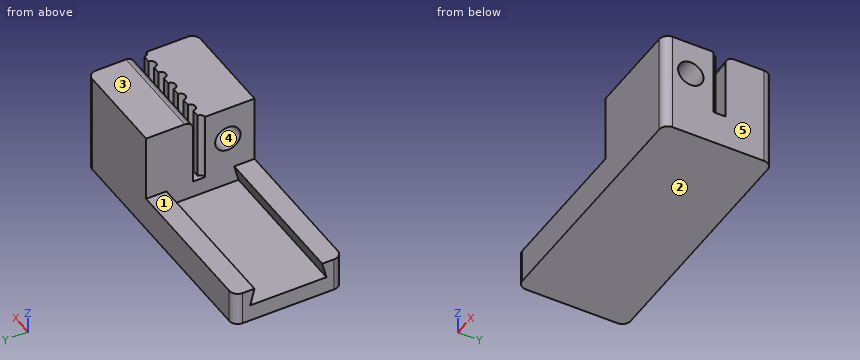
```python
from build123d import *

# Parameters (mm, degrees)
BOSS_EXTRUDE1_DEPTH = 12
CUT_EXTRUDE1_DEPTH  = 8
FILLET1_R           = 1
CUT_EXTRUDE3_DEPTH  = 18
SKETCH6_R           = 1.5
CUT_EXTRUDE2_DEPTH  = 12


with BuildPart() as part:
    # Sketch4 → Boss-Extrude1 (new body)
    with BuildSketch(Plane.XY):
        with BuildLine():
            Line((12, 1.1), (12, 11.9))
            ThreePointArc((12, 11.9), (11.707106781, 12.607106781), (11, 12.9))
            Line((11, 12.9), (-17, 12.9))
            ThreePointArc((-17, 12.9), (-17.707106781, 12.607106781), (-18, 11.9))
            Line((-18, 11.9), (-18, 1.1))
            ThreePointArc((-18, 1.1), (-17.707106781, 0.392893219), (-17, 0.1))
            Line((-17, 0.1), (11, 0.1))
            ThreePointArc((11, 0.1), (11.707106781, 0.392893219), (12, 1.1))
        make_face()
    extrude(amount=BOSS_EXTRUDE1_DEPTH)

    # Sketch5 → Cut-Extrude1 (cut)
    with BuildSketch(Plane.XY.offset(12)):
        with BuildLine():
            Line((11.445, 6.5), (10.555, 6.5))
            ThreePointArc((10.555, 6.5), (10, 5.945), (9.445, 6.5))
            Line((9.445, 6.5), (8.555, 6.5))
            ThreePointArc((8.555, 6.5), (8, 5.945), (7.445, 6.5))
            Line((7.445, 6.5), (6.555, 6.5))
            ThreePointArc((6.555, 6.5), (6, 5.945), (5.445, 6.5))
            Line((5.445, 6.5), (4.555, 6.5))
            ThreePointArc((4.555, 6.5), (4, 5.945), (3.445, 6.5))
            Line((3.445, 6.5), (2.555, 6.5))
            ThreePointArc((2.555, 6.5), (2, 5.945), (1.445, 6.5))
            Line((1.445, 6.5), (0.555, 6.5))
            ThreePointArc((0.555, 6.5), (0.392444264, 6.107555736), (0, 5.945))
            Line((0, 5.945), (0, 7.345))
            Line((0, 7.345), (12, 7.345))
            Line((12, 7.345), (12, 5.945))
            ThreePointArc((12, 5.945), (11.607555736, 6.107555736), (11.445, 6.5))
        make_face()
    extrude(amount=-CUT_EXTRUDE1_DEPTH, mode=Mode.SUBTRACT)

    # Fillet1
    fillet1_edges = [part.edges().sort_by_distance(p)[0] for p in [
        (6, 7.345, 12),
    ]]
    fillet(fillet1_edges, radius=FILLET1_R)

    # Sketch7 → Cut-Extrude3 (cut)
    with BuildSketch(Plane.ZY.offset(18)):
        Polygon((4, 10.5), (4, 12.9), (12, 12.9), (12, 0.1), (4, 0.1), (4, 2.5), (2, 2), (2, 11), align=None)
    extrude(amount=-CUT_EXTRUDE3_DEPTH, mode=Mode.SUBTRACT)

    # Sketch6 → Cut-Extrude2 (cut)
    with BuildSketch(Plane.ZY.offset(-12)):
        with Locations((8, 3.25)):
            Circle(SKETCH6_R)
    extrude(amount=CUT_EXTRUDE2_DEPTH, mode=Mode.SUBTRACT)


solid = part.part
```
Model file for the job. Use its own axes, mm. Face numbers are marked on the shaded views. A direction names the side the tool comes from. Give positions to 0.01 mm unless a question says otherwise; leave off trailing zeros. Order: outer loops, then holes, each group sorted by start corner. A loop starts at its lowest first (then second) coordinate and runs counter-clockwise, first axis right, second up.
1) Mould opens along Z. For the marked faces 3, 4 and 5 say: +Z half, -Z half, draft (parallel to the pull), parting line (faces both ways), or undercut.
2) Saw through at D-D, the plane x = 4. Write the cut outline in (y, z) (3 decimals).
3) Saw through at A-A, the plane y = 3.25. Write the cut outline in (x, z), then the cut area to 3 significant figures.
4) Saw through at C-C, the plane z = 10.5. Write the cut outline in (x, y) (3 decimals).
5) Pin check, flat tips, straight feed: pin 1 (3.5 mm diameter, centred on y = 3.25, z = 8, fed in from -X); pin 2 (2.5 mm diameter, centred on x = -9, y = 1.5, fed in from +Z); pin 3 (3 mm diameter, centred on x = -1.5, y = 8, fed in from -Z). Stop position of each tip, or through.
6) Wall check: probe 1 along Y at (x, z) = (6, 8) (3 decimals); probe 2 along Z at (x, y) = (9.5, 8.25). Give the ranges that are in metal, low to high.
7) Saw through at B-B, the plane z = 8. Write the cut outline in (x, y) (3 decimals), then the cut area to 3 significant figures.
8) 3-axis set-ups, long thin cutter, end or side, ignore diameter. For the marked faces 1 and 2: which of +Z, -Z, +X, -X, +Y, -Y reach the whole face in a straight line?
Computed:
1. face 3: +Z half
1. face 4: undercut
1. face 5: draft
2. outline: (0.1, 0) - (12.9, 0) - (12.9, 12) - (8.345, 12) arc R1 ccw to (7.345, 11) - (7.345, 4) - (5.945, 4) - (5.945, 12) - (0.1, 12) - close; hole circle Ø3 at (3.25, 8)
3. outline: (-18, 0) - (12, 0) - (12, 6.5) - (0, 6.5) - (0, 2) - (-18, 2) - close; (0, 9.5) - (12, 9.5) - (12, 12) - (0, 12) - close
3. area: 144 mm2
4. outline: (0, 0.1) - (11, 0.1) arc R1 ccw to (12, 1.1) - (12, 5.945) arc R0.555 cw to (11.445, 6.5) - (10.555, 6.5) arc R0.555 cw to (9.445, 6.5) - (8.555, 6.5) arc R0.555 cw to (7.445, 6.5) - (6.555, 6.5) arc R0.555 cw to (5.445, 6.5) - (4.555, 6.5) arc R0.555 cw to (3.445, 6.5) - (2.555, 6.5) arc R0.555 cw to (1.445, 6.5) - (0.555, 6.5) arc R0.555 cw to (0, 5.945) - close; (0, 7.345) - (12, 7.345) - (12, 11.9) arc R1 ccw to (11, 12.9) - (0, 12.9) - close
5. pin 1: stops at x = 0
5. pin 2: stops at z = 4
5. pin 3: stops at z = 0
6. probe 1: y = 0.1 to 1.75, 4.75 to 5.945, 7.345 to 12.9
6. probe 2: z = 0 to 12
7. outline: (0, 0.1) - (11, 0.1) arc R1 ccw to (12, 1.1) - (12, 1.75) - (0, 1.75) - close; (0, 4.75) - (12, 4.75) - (12, 5.945) arc R0.555 cw to (11.445, 6.5) - (10.555, 6.5) arc R0.555 cw to (9.445, 6.5) - (8.555, 6.5) arc R0.555 cw to (7.445, 6.5) - (6.555, 6.5) arc R0.555 cw to (5.445, 6.5) - (4.555, 6.5) arc R0.555 cw to (3.445, 6.5) - (2.555, 6.5) arc R0.555 cw to (1.445, 6.5) - (0.555, 6.5) arc R0.555 cw to (0, 5.945) - close; (0, 7.345) - (12, 7.345) - (12, 11.9) arc R1 ccw to (11, 12.9) - (0, 12.9) - close
7. area: 104 mm2
8. face 1: +Z, -X, +Y, -Y
8. face 2: -Z, +X, -X, +Y, -Y
